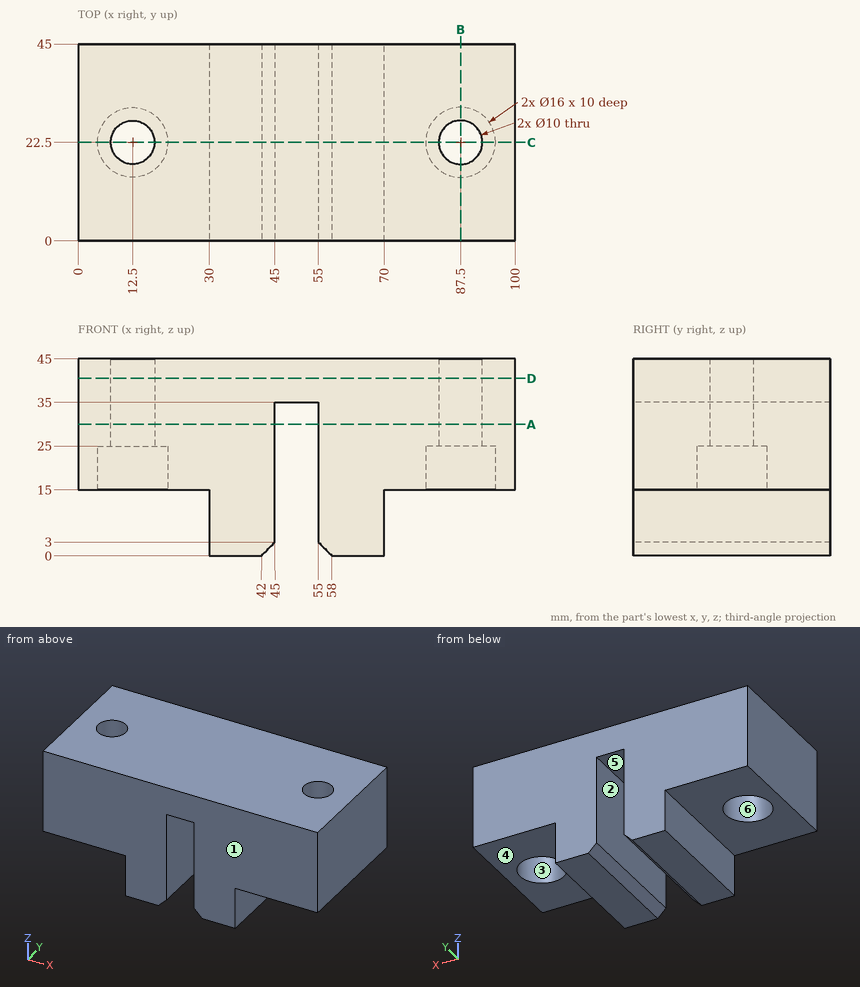
Could you check a few things on this drawing? It's one solid part, dimensions in mm from its lowest x, y, z. A direction names the side the tool comes from. Give positions to 0.01 mm unless a question says otherwise; leave off trailing zeros. Order: outer loops, then holes, each group sorted by start corner. A loop starts at its lowest first (then second) coordinate and runs counter-clockwise, first axis right, second up. Notation, with made-up numbers: (-3, 69) -> (11, 69) arc R26 ccw to (11, 107) -> close; hole circle Ø6 at (10.25, -35). An arc over 180 degrees is marked (long way). Answer in a Markdown table with one row per item. Add a question column.
Item 1: For the marked faces 4, 5 and 6, which set-ups out of +Z, -Z, +X, -X, +Y, -Y let a thin tool reach every point of the face, with its end or its side?
Item 2: Imagine slicing it at B-B (x = 87.5). List the corners of the cut face in (y, z) for me, and give its area (3 significant figures).
Item 3: I'm going to push flat-ended pins straight in: P1, Ø5, axis at x = 49, y = 27, coming from the -Z side; P2, Ø8, axis at y = 19, z = 13.5, coming from the -X side; P3, Ø18.5, axis at x = 87.5, y = 22.5, coming from the -Z side; P4, Ø7.5, axis at y = 33.5, z = 8, coming from the +X side. Where does each tip first touch, or does it pass through?
Item 4: We'd pull the mould along Y, two halves only. Please class the marked faces 1, 2 and 3: pulls with the +Y half, pulls with the -Y half, needs draft (parallel to the pull), parting line crosses it, or undercut.
Item 5: Imagine slicing it at D-D (z = 40.5). List the corners of the cut face in (x, y) for me, and give its area (3 significant figures).
Item 6: Imagine slicing it at C-C (y = 22.5). Count the separate pieces of the cut face and the enclosed holes in it, and give its area (3 significant figures).
Item 7: Imagine slicing it at A-A (z = 30). List the corners of the cut face in (x, y) for me.
Item 8: Please list where these lines run through material, in increasing order: probe 1 along X at (y, z) = (22, 22); probe 2 along X at (y, z) = (27, 31); probe 3 along X at (y, z) = (10.5, 17).
Result:
| question | item | result |
|---|---|---|
| 1 | face 4 | -Z, +X, +Y, -Y |
| 1 | face 5 | -Z, +Y, -Y |
| 1 | face 6 | -Z |
| 2 | outline | (0, 15) -> (14.5, 15) -> (14.5, 25) -> (17.5, 25) -> (17.5, 45) -> (0, 45) -> close; (27.5, 25) -> (30.5, 25) -> (30.5, 15) -> (45, 15) -> (45, 45) -> (27.5, 45) -> close |
| 2 | area | 990 mm2 |
| 3 | P1 | z = 35 |
| 3 | P2 | x = 0 |
| 3 | P3 | z = 15 |
| 3 | P4 | x = 70 |
| 4 | face 1 | pulls with the -Y half |
| 4 | face 2 | needs draft |
| 4 | face 3 | undercut |
| 5 | outline | (0, 0) -> (100, 0) -> (100, 45) -> (0, 45) -> close; hole circle Ø10 at (12.5, 22.5); hole circle Ø10 at (87.5, 22.5) |
| 5 | area | 4,340 mm2 |
| 6 | separate pieces | 3 |
| 6 | enclosed holes | 0 |
| 6 | area | 2,520 mm2 |
| 7 | outline | (0, 0) -> (45, 0) -> (45, 45) -> (0, 45) -> close; (55, 0) -> (100, 0) -> (100, 45) -> (55, 45) -> close; hole circle Ø10 at (12.5, 22.5); hole circle Ø10 at (87.5, 22.5) |
| 8 | probe 1 | 0 to 4.52, 20.48 to 45, 55 to 79.52, 95.48 to 100 |
| 8 | probe 2 | 0 to 10.32, 14.68 to 45, 55 to 85.32, 89.68 to 100 |
| 8 | probe 3 | 0 to 45, 55 to 100 |
